```python
from build123d import *

# Parameters (mm, degrees)
SKETCH1_R                                            = 12.5
BOSS_EXTRUDE1_DEPTH                                  = 19
CUT_EXTRUDE1_REACH                                   = 27.952
SKETCH3_R                                            = 6.975
CUT_EXTRUDE2_DEPTH                                   = 6.54
SKETCH5_R                                            = 0.5
CUT_EXTRUDE4_DEPTH                                   = 17.5
CUT_EXTRUDE5_DEPTH                                   = 15
REFRENTADO_PARA_TORNILLO_TAP_N_CON_CABEZ_D           = 3.91
REFRENTADO_PARA_TORNILLO_TAP_N_CON_CABEZ_CBORE_D     = 6.5
REFRENTADO_PARA_TORNILLO_TAP_N_CON_CABEZ_CBORE_DEPTH = 8
CHAFL_N1_SIZE                                        = 0.5
DODANIE_WYCI_GNI_CIE1_START                          = -10
DODANIE_WYCI_GNI_CIE1_DEPTH                          = 10


with BuildPart() as part:
    # Sketch1 → Boss-Extrude1 (new body)
    with BuildSketch(Plane(origin=(0, 0, 0), x_dir=(0, 0, -1), z_dir=(1, 0, 0))):
        Circle(SKETCH1_R)
    extrude(amount=BOSS_EXTRUDE1_DEPTH)

    # Sketch3 → Cut-Extrude1 (cut, up to next)
    with BuildSketch(Plane.ZY, mode=Mode.PRIVATE) as cut_extrude1_sk1:
        Circle(SKETCH3_R)
    cut_extrude1_tool1 = extrude(cut_extrude1_sk1.sketch, amount=-CUT_EXTRUDE1_REACH, mode=Mode.PRIVATE) & part.part
    add(cut_extrude1_tool1.solids().sort_by_distance((0, 0, 0))[0], mode=Mode.SUBTRACT)

    # Sketch2 → Cut-Extrude2 (cut)
    with BuildSketch(Plane.ZY):
        with BuildLine():
            Line((6.876343086, 1.168987069), (6.876343086, -1.168987069))
            ThreePointArc((6.876343086, -1.168987069), (0, -29.5), (-6.876343086, -1.168987069))
            Line((-6.876343086, -1.168987069), (-6.876343086, 1.168987069))
            ThreePointArc((-6.876343086, 1.168987069), (0, 29.5), (6.876343086, 1.168987069))
        make_face()
    extrude(amount=-CUT_EXTRUDE2_DEPTH, mode=Mode.SUBTRACT)

    # Sketch5 → Cut-Revolve1 (revolve, cut)
    with BuildSketch(Plane(origin=(0, 0, 0), x_dir=(-1, 0, 0), z_dir=(0, -1, 0)), mode=Mode.PRIVATE) as cut_revolve1_sk:
        with Locations((-3.64, 12.8)):
            Circle(SKETCH5_R)
    revolve(cut_revolve1_sk.sketch.rotate(Axis((19, 0, 0), (-1, 0, 0)), 202.975957279), axis=Axis((19, 0, 0), (-1, 0, 0)), mode=Mode.SUBTRACT)

    # Sketch6 → Cut-Extrude4 (cut, symmetric)
    with BuildSketch(Plane(origin=(0, 0, 0), x_dir=(1, 0, 0), z_dir=(0, 1, 0))):
        with BuildLine():
            Line((9, 14.85), (9, -1.85))
            ThreePointArc((9, -1.85), (8.5, -2.35), (8, -1.85))
            Line((8, -1.85), (8, 14.85))
            Line((8, 14.85), (9, 14.85))
        make_face()
    extrude(amount=CUT_EXTRUDE4_DEPTH, both=True, mode=Mode.SUBTRACT)

    # Sketch9 → Cut-Extrude5 (cut)
    with BuildSketch(Plane(origin=(0, 0, 0), x_dir=(1, 0, 0), z_dir=(0, 1, 0))):
        with BuildLine():
            Line((8.5, -1.35), (27.798520731, -1.35))
            ThreePointArc((27.798520731, -1.35), (28.298520731, -1.85), (27.798520731, -2.35))
            Line((27.798520731, -2.35), (8.5, -2.35))
            ThreePointArc((8.5, -2.35), (8, -1.85), (8.5, -1.35))
        make_face()
    extrude(amount=-CUT_EXTRUDE5_DEPTH, mode=Mode.SUBTRACT)

    # Refrentado para tornillo tapón con cabeza de clavija de M2.51 (through all)
    with Locations(Plane(origin=(0, 0, -13.65), x_dir=(1, 0, 0), z_dir=(0, 0, -1))):
        with Locations((14, 7.426886175)):
            CounterBoreHole(REFRENTADO_PARA_TORNILLO_TAP_N_CON_CABEZ_D / 2, REFRENTADO_PARA_TORNILLO_TAP_N_CON_CABEZ_CBORE_D / 2, REFRENTADO_PARA_TORNILLO_TAP_N_CON_CABEZ_CBORE_DEPTH)

    # Chaflán1
    chafl_n1_edges = [part.edges().sort_by_distance(p)[0] for p in [
        (0, 0, 12.5),
        (0, 0, -12.5),
        (19, 9.633924434, 7.964766161),
    ]]
    chamfer(chafl_n1_edges, length=CHAFL_N1_SIZE)

    # Szkic1 → Dodanie-wyciągnięcie1 (add)
    with BuildSketch(Plane(origin=(19, 0, 0), x_dir=(0, 0, -1), z_dir=(1, 0, 0)).offset(DODANIE_WYCI_GNI_CIE1_START)):
        with BuildLine():
            Line((-2.35, -6.567200697), (-2.35, -2.134976581))
            ThreePointArc((-2.35, -2.134976581), (1.88651169, 2.553761665), (-1.35, -2.873695356))
            Line((-1.35, -2.873695356), (-1.35, -6.843107847))
            ThreePointArc((-1.35, -6.843107847), (1.855136434, 6.723770803), (-2.35, -6.567200697))
        make_face()
    extrude(amount=DODANIE_WYCI_GNI_CIE1_DEPTH)


solid = part.part
```
Can you work these out from the model? Positions are in its coordinate system, mm. A direction names the side the tool comes from. Give positions to 0.01 mm unless a question says otherwise; leave off trailing zeros. Write each loop counter-clockwise with the first axis right and the second up, starting at its lowest first coordinate (ties: lowest second). Pieces come first, ordered by that corner, then holes. Notation, with made-up numbers: (-4, -6) - (8, -6) arc R15 cw to (8, 20) - close; hole circle Ø3 at (26, 27). An arc over 180 degrees is marked (long way). Write item = value, one per line. Start each with the question number.
1. Imagine slicing it at B-B (x = 2). Please give me the cut outline in (y, z) (3 decimals).
2. Please list where these lines run through material, in increasing order: line 1 (X direction, y = -6, z = -4.5); line 2 (Y direction, x = 15.5, z = 0) (3 decimals); line 3 (X direction, y = -9, z = -6.5).
3. For pin 1 (9 mm diameter, centred on y = -7, z = 1.5, fed in from -X); pin 2 (10 mm diameter, centred on y = 0, z = 0, fed in from -X); pin 3 (5 mm diameter, centred on x = 14, y = -7.43, fed in from -Z); pin 4 (8.5 mm diameter, centred on y = 0, z = 0, fed in from +X), each with a flat end and sliding along its axis, tell me the tip position at first contact or that it passes through.
4. Imagine slicing it at A-A (z = 0). Please give me the cut outline in (x, y) (3 decimals).
5. On a 3-axis mill with a long thin cutter (end or side, diameter ignored), from which of +Z, -Z, +X, -X, +Y, -Y can I reach the whole of each face in a straight line? I mean faces 5 (the face through (6.54, 8, 0)), 6 (the face through (14.424, -5.518, 6.857)), 7 (the face through (8, 0, -8)), 8 (the face through (13.295, -4.254, -8.077)), 9 (the face through (13.97, -6.79, -1.6)). Say none if no direction works.
6. Thinking about a two-plate mould opening in Y: for faces 1 (the face through (6.54, -8, 0)), 2 (the face through (1.9, 0.1, 12.5)), 3 (the face through (6.146, -0.911, 6.915)), 4 (the face through (9, 0, -5)), which applies, released by +Y, released by -Y, zero draft, split by the parting line, or undercut?
7. Imagine slicing it at C-C (x = 14). Count the separate pieces of the cut face and the enclosed holes in it, and give its area (3 significant figures).
Worked answers:
q1.outline = (-4.879, -11.508) arc R12.5 ccw to (4.879, -11.508) arc R15 cw to (1.169, -6.876) arc R6.975 cw to (-1.169, -6.876) arc R15 cw to start; (-4.879, 11.508) arc R15 cw to (-1.169, 6.876) arc R6.975 cw to (1.169, 6.876) arc R15 cw to (4.879, 11.508) arc R12.5 ccw to start
q2.line_1 = 6.54 to 8, 9 to 12.66, 15.34 to 19
q2.line_2 = -12.5 to -8.681, -6.975 to -3.175, 3.175 to 12.5
q2.line_3 = 6.54 to 8, 9 to 11.16, 16.84 to 19
q3.pin_1 = 6.54
q3.pin_2 = 9
q3.pin_3 = -5.65
q3.pin_4 = 19
q4.outline = (6.54, -12.5) - (8, -12.5) - (8, -6.975) - (6.54, -6.975) - close; (6.54, 6.975) - (8, 6.975) - (8, 12.5) - (6.54, 12.5) - close; (9, -12.5) - (18.5, -12.5) - (19, -12) - (19, -3.175) - (9, -3.175) - close; (9, 3.175) - (19, 3.175) - (19, 12) - (18.5, 12.5) - (9, 12.5) - close; hole (12.098, -6.975) arc R1.955 ccw (long way) to (15.902, -6.975) - close
q5.face_5 = -X, +Y
q5.face_6 = +Z
q5.face_7 = -Z, +Y, -Y
q5.face_8 = -Z
q5.face_9 = none
q6.face_1 = zero draft
q6.face_2 = split by the parting line
q6.face_3 = undercut
q6.face_4 = undercut
q7.separate_pieces = 3
q7.enclosed_holes = 0
q7.area = 373 mm2
